from build123d import *

# Parameters (mm, degrees)
F0_W        = 40
F0_H        = 50
F0_R        = 2
F1_DEPTH    = 6
F2_R        = 13.6797776514
F3_DEPTH    = 100
F4_R        = 23.0640267833
F5_DEPTH    = 10
F6_S5_R     = 13.6797776514
F6_T6_DEPTH = 34
F7_R        = 3
F8_SIZE     = 5.08
F9_SIZE     = 2.5


# Not quite as in the source:
# - a fillet or chamfer that OpenCascade refuses, or shapes differently, is made with other operations: its cross-section is extruded or revolved along the edge and cut away or added


with BuildPart() as f1:
    # F0 (on Top) → F1 (new body)
    with BuildSketch(Plane.XY):
        with Locations((20, 25)):
            Rectangle(F0_W, F0_H)
        with Locations((20, 5)):
            Circle(F0_R, mode=Mode.SUBTRACT)
        with Locations((20, 45)):
            Circle(F0_R, mode=Mode.SUBTRACT)
    extrude(amount=F1_DEPTH)

    # F2 (on face) → F3 (join)
    with BuildSketch(Plane.XY.offset(6)):
        with Locations((20, 24.1802949458)):
            Circle(F2_R)
    extrude(amount=F3_DEPTH)

    # F4 (on face) → F5 (join)
    with BuildSketch(Plane.XY.offset(106)):
        with Locations((20, 24.1802949458)):
            Circle(F4_R)
    extrude(amount=F5_DEPTH)

    # F6: chamfer of 10 on 1 edges, made by hand


with BuildPart() as f6_tool2:
    # F6_s3 → F6_t4 (revolve)
    with BuildSketch(Plane.XZ.offset(-24.1802949458)):
        Polygon((43.0640267833, 116), (33.0640267833, 106), (43.0640267833, 106), align=None)
    revolve(axis=Axis((20, 24.1802949458, 106), (0, 0, 1)))

    # F6_s5 → F6_t6 (cut, symmetric)
    with BuildSketch(Plane.XY.offset(111)):
        with Locations((20, 24.1802949458)):
            Circle(F6_S5_R)
    extrude(amount=F6_T6_DEPTH, both=True, mode=Mode.SUBTRACT)


with BuildPart() as f1_1:
    add(f1.part)

    # F6_t1: cut F6_tool2
    add(f6_tool2.part, mode=Mode.SUBTRACT)

    # F7
    f7_edges = [f1_1.edges().sort_by_distance(p)[0] for p in [
        (-3.064027, 24.180295, 116),
    ]]
    fillet(f7_edges, radius=F7_R)

    # F8
    f8_edges = [f1_1.edges().sort_by_distance(p)[0] for p in [
        (40, 0, 3),
        (40, 50, 3),
        (0, 50, 3),
        (0, 0, 3),
    ]]
    chamfer(f8_edges, length=F8_SIZE)

    # F9
    f9_edges = [f1_1.edges().sort_by_distance(p)[0] for p in [
        (18, 5, 6),
        (18, 45, 6),
    ]]
    chamfer(f9_edges, length=F9_SIZE)


solid = f1_1.part
Work out the finished part from the listing and answer in its coordinate system (mm). A direction names the side the tool comes from. Coordinates: 2 decimals unless noted, no trailing zeros. Write each loop counter-clockwise with the first axis right and the second up, starting at its lowest first coordinate (ties: lowest second). Pieces come first, ordered by that corner, then holes.
1. For faces 4 (the conical face through (18.32, 3.71, 3.62)), 5 (the cylindrical face through (18, 5, 2)), 6 (the flat face through (37.5, 2.58, 2.96)), determine the directions among +Z, -Z, +X, -X, +Y, -Y from which every point of the face is accessible in a straight line to the end or side of a thin tool.
Results list:
face 4: none
face 5: -Z
face 6: +Z, -Z, +X, -Y
2. Consider line 1 along Y through (x, z) = (20, 1); line 2 along Z through (x, y) = (31, 47); line 3 along Z through (x, y) = (8.5, 38). Determine where each line is inside the solid, lowest interval first.
Results list:
line 1: y = 0 to 3, 7 to 43, 47 to 50
line 2: z = 0 to 6
line 3: z = 0 to 6, 110.92 to 115.08
3. The part is cut by section A-A, the plane x = 20. Write down the section's boundary in (y, z), and give its area (3 significant figures).
Results list:
outline: (0, 0) - (3, 0) - (3, 3.5) - (0.5, 6) - (0, 6) - close; (6.24, 110.88) - (10.5, 106.62) - (10.5, 6) - (9.5, 6) - (7, 3.5) - (7, 0) - (43, 0) - (43, 3.5) - (40.5, 6) - (37.86, 6) - (37.86, 106.62) - (42.12, 110.88) arc R3 ccw to (40, 116) - (8.36, 116) arc R3 ccw to start; (47, 0) - (50, 0) - (50, 6) - (49.5, 6) - (47, 3.5) - close
area: 3,310 mm2
4. For a pull along Z with two mould halves and no side action, classify faces 1 (the flat face through (20, 24, 116)), 2 (the cylindrical face through (26.312, 12.044, 55.604)), 3 (the flat face through (37.5, 47.42, 2.96)) as +Z half, -Z half, draft (parallel to the pull), parting line (faces both ways), or undercut.
Results list:
face 1: +Z half
face 2: undercut
face 3: draft
5. Flat-ended cylindrical pins translate along their axes: pin 1 (4 mm diameter, centred on x = 10, z = 35.5, fed in from +Y); pin 2 (6.5 mm diameter, centred on x = 20, y = 5, fed in from -Z); pin 3 (6 mm diameter, centred on x = 11, y = 42, fed in from +Z); pin 4 (6 mm diameter, centred on x = 29, z = 85, fed in from -Y). Find the tip coordinate at first contact, or state that the pin passes through.
Results list:
pin 1: stops at y = 35.28
pin 2: stops at z = 0
pin 3: stops at z = 115.77
pin 4: stops at y = 11.89
6. The part is cut by section B-B, the plane z = 47.5. Write down the section's boundary in (x, y), and give its area (3 significant figures).
Results list:
outline: circle Ø27.36 at (20, 24.18)
area: 588 mm2
